Build history of the part. All positions in model axes, mm. A direction names the side the tool comes from. Give positions to 0.01 mm unless a question says otherwise; leave off trailing zeros. Order: outer loops, then holes, each group sorted by start corner. A loop starts at its lowest first (then second) coordinate and runs counter-clockwise, first axis right, second up. Notation, with made-up numbers: (-27, 0) - (-1, 0) arc R22 ccw to (-1, 33) - close; hole circle Ø11 at (43.5, 43.5). An arc over 180 degrees is marked (long way). Answer in a Markdown table with one row per item.
```python
from build123d import *

# Parameters (mm, degrees)
CYLINDER003_R            = 2.65
CYLINDER003_DEPTH        = 9
CLONE009_PLACEMENT_ANGLE = 90
BOX002_W                 = 12
BOX002_H                 = 24
BOX002_DEPTH             = 8
FILLET_R                 = 2
CYLINDER002_R            = 0.925
CYLINDER002_DEPTH        = 7
CYLINDER001_R            = 3
CYLINDER001_DEPTH        = 7
SKETCH002_R              = 1.65
EXTRUDE002_DEPTH         = 3
CLONE010_PLACEMENT_ANGLE = 90


with BuildPart() as insert001:
    # Cylinder003 → Cylinder003 (new body)
    with BuildSketch(Plane(origin=(24, -35, 3), x_dir=(0, 0, 1), z_dir=(-1, 0, 0))):
        Circle(CYLINDER003_R)
    extrude(amount=CYLINDER003_DEPTH)


with BuildPart() as insert002:
    # Clone006 base: copy of insert001
    add(insert001.part)


with BuildPart() as insert002_1:
    # Clone006 placement: moved
    add(insert002.part.moved(Location((0, -16, 0))))


with BuildPart() as obj1:
    # Fusion002 base: copy of insert001
    add(insert001.part)

    # Fusion002: union insert002
    add(insert002_1.part)


with BuildPart() as obj1_1:
    # Fusion002 placement: moved
    add(obj1.part.moved(Location((0, 0, -3))))


with BuildPart() as insertsfusion003:
    # Clone009 base: copy of obj1
    add(obj1_1.part)


with BuildPart() as insertsfusion003_1:
    # Clone009 placement: moved
    add(insertsfusion003.part.moved(Location((0, 50, 62))).rotate(Axis((0, 50, 62), (1, 0, 0)), CLONE009_PLACEMENT_ANGLE))

    # Fusion003: union obj1
    add(obj1_1.part)


with BuildPart() as obj2:
    # Box002 → Box002 (new body)
    with BuildSketch(Plane(origin=(15, -55, -1), x_dir=(1, 0, 0), z_dir=(0, 0, 1))):
        with Locations((6, 12)):
            Rectangle(BOX002_W, BOX002_H)
    extrude(amount=BOX002_DEPTH)

    # Fillet
    fillet_edges = [obj2.edges().sort_by_distance(p)[0] for p in [
        (21, -55, -1),
        (21, -55, 7),
        (21, -31, -1),
        (21, -31, 7),
    ]]
    fillet(fillet_edges, radius=FILLET_R)


with BuildPart() as obj2_1:
    # Fillet placement: moved
    add(obj2.part.moved(Location((0, 0, -3))))


with BuildPart() as hole002:
    # Cylinder002 → Cylinder002 (new body)
    with BuildSketch(Plane(origin=(27, -16, 0), x_dir=(0, 0, 1), z_dir=(-1, 0, 0))):
        Circle(CYLINDER002_R)
    extrude(amount=CYLINDER002_DEPTH)


with BuildPart() as hole003:
    # Clone003 base: copy of hole002
    add(hole002.part)


with BuildPart() as hole003_1:
    # Clone003 placement: moved
    add(hole003.part.moved(Location((0, 0, 36))))


with BuildPart() as hole004:
    # Clone004 base: copy of hole003
    add(hole003_1.part)


with BuildPart() as hole004_1:
    # Clone004 placement: moved
    add(hole004.part.moved(Location((0, 56, -36))))


with BuildPart() as hole005:
    # Clone005 base: copy of hole004
    add(hole004_1.part)


with BuildPart() as hole005_1:
    # Clone005 placement: moved
    add(hole005.part.moved(Location((0, 0, 36))))


with BuildPart() as holesfusion001:
    # Fusion base: copy of hole002
    add(hole002.part)

    # Fusion: union hole003, hole004, hole005
    add(hole003_1.part)
    add(hole004_1.part)
    add(hole005_1.part)


with BuildPart() as attach001:
    # Cylinder001 → Cylinder001 (new body)
    with BuildSketch(Plane(origin=(27, 40, 0), x_dir=(0, 0, 1), z_dir=(-1, 0, 0))):
        Circle(CYLINDER001_R)
    extrude(amount=CYLINDER001_DEPTH)


with BuildPart() as attach002:
    # Clone base: copy of attach001
    add(attach001.part)


with BuildPart() as attach002_1:
    # Clone placement: moved
    add(attach002.part.moved(Location((0, 0, 36))))


with BuildPart() as attach003:
    # Clone001 base: copy of attach002
    add(attach002_1.part)


with BuildPart() as attach003_1:
    # Clone001 placement: moved
    add(attach003.part.moved(Location((0, -56, -36))))


with BuildPart() as attach004:
    # Clone002 base: copy of attach003
    add(attach003_1.part)


with BuildPart() as attach004_1:
    # Clone002 placement: moved
    add(attach004.part.moved(Location((0, 0, 36))))


with BuildPart() as obj3:
    # Sketch002 (on Face5 of Extrude001) → Extrude002 (new body)
    with BuildSketch(Plane.YZ.offset(27)):
        with BuildLine():
            Line((-21.840834, 24.960582), (-53.988857, 12.50779))
            ThreePointArc((-53.988857, 12.50779), (-56.115528, 9.746452), (-54.651077, 6.583683))
            add(Edge.make_bspline(
                [(-54.651077, 6.583683), (-53.010517, 3.198744), (-52.696371, 2.249369), (-51.549184, 1.787077), (-52.006912, 2.204484), (-45.648689, -0.330521), (-21.747141, 0.945049), (-21.747141, 0.945049)],
                knots=[0, 0, 0, 0, 0.2, 0.4, 0.6, 0.8, 1, 1, 1, 1], degree=3))
            ThreePointArc((-21.747141, 0.945049), (-20.257929, 0.297113), (-19.355012, -1.052819))
            ThreePointArc((-19.355012, -1.052819), (-18.192035, -2.749458), (-16.278951, -3.505242))
            Line((-16.278951, -3.505242), (38.983907, -3.505242))
            ThreePointArc((38.983907, -3.505242), (40.694219, -3.582907), (42.251751, -2.872069))
            Line((42.251751, -2.872069), (47.13375, -1.117604))
            ThreePointArc((47.13375, -1.117604), (49.660876, -0.395307), (51.055069, 1.832764))
            Line((51.055069, 1.832764), (49.885408, 38.110058))
            ThreePointArc((49.885408, 38.110058), (50.422789, 40.457526), (52.04587, 42.236569))
            ThreePointArc((52.04587, 42.236569), (53.292041, 46.426402), (49.345321, 48.305506))
            Line((49.345321, 48.305506), (31.159741, 40.29296))
            ThreePointArc((31.159741, 40.29296), (28.834741, 39.544977), (26.405518, 39.292031))
            Line((26.405518, 39.292031), (-15.565081, 39.292031))
            ThreePointArc((-15.565081, 39.292031), (-18.351405, 38.137898), (-19.505538, 35.351575))
            Line((-19.505538, 35.351575), (-19.505538, 28.369553))
            ThreePointArc((-19.505538, 28.369553), (-20.14535, 26.303476), (-21.840834, 24.960582))
        make_face()
        with Locations((-52.774566, 9.372986)):
            Circle(SKETCH002_R, mode=Mode.SUBTRACT)
        with Locations((50.220626, 45.059686)):
            Circle(SKETCH002_R, mode=Mode.SUBTRACT)
        with Locations((46.966619, 2.182986)):
            Circle(SKETCH002_R, mode=Mode.SUBTRACT)
        with BuildLine():
            ThreePointArc((-42.901854, 12.302255), (-43.81194, 10.903698), (-42.6099, 9.746408))
            Line((-42.6099, 9.746408), (41.00829, 3.39546))
            ThreePointArc((41.00829, 3.39546), (44.698125, 5.221862), (46.188436, 9.059779))
            Line((46.188436, 9.059779), (46.188436, 30.650335))
            ThreePointArc((46.188436, 30.650335), (45.602859, 32.064042), (44.189151, 32.649619))
            Line((44.189151, 32.649619), (13.812123, 32.649619))
            Line((13.812123, 32.649619), (-11.694611, 34.281909))
            ThreePointArc((-11.694611, 34.281909), (-13.16559, 33.801037), (-13.900901, 32.439297))
            ThreePointArc((-13.900901, 32.439297), (-13.932701, 32.072334), (-13.943313, 31.704149))
            Line((-13.943313, 31.704149), (-13.943313, 26.615805))
            ThreePointArc((-13.943313, 26.615805), (-14.202233, 24.971619), (-14.953931, 23.48658))
            Line((-14.953931, 23.48658), (-15.353167, 22.932962))
            ThreePointArc((-15.353167, 22.932962), (-16.05756, 22.212579), (-16.942805, 21.731473))
            Line((-16.942805, 21.731473), (-42.901854, 12.302255))
        make_face(mode=Mode.SUBTRACT)
    extrude(amount=-EXTRUDE002_DEPTH)

    # Fusion001: union attach004, attach003, attach002, attach001
    add(attach004_1.part)
    add(attach003_1.part)
    add(attach002_1.part)
    add(attach001.part)

    # Cut001: cut holesFusion001
    add(holesfusion001.part, mode=Mode.SUBTRACT)


with BuildPart() as obj4:
    # Clone010 base: copy of obj2
    add(obj2_1.part)


with BuildPart() as obj4_1:
    # Clone010 placement: moved
    add(obj4.part.moved(Location((0, 50, 62))).rotate(Axis((0, 50, 62), (1, 0, 0)), CLONE010_PLACEMENT_ANGLE))

    # Fusion004: union obj2, obj3
    add(obj2_1.part)
    add(obj3.part)

    # Cut002: cut insertsFusion003
    add(insertsfusion003_1.part, mode=Mode.SUBTRACT)


solid = obj4_1.part
```
1. Two-plate mould, pull along Z, no slides. Class faces 6 (the face through (26, -13.943, 29)), 7 (the face through (25.521, -20.128, 26.329)), 8 (the face through (21.08, -31.57, -3.4)): +Z half, -Z half, draft (parallel to the pull), parting line (faces both ways), or undercut.
Check result:
| item | result |
|---|---|
| face 6 | undercut |
| face 7 | +Z half |
| face 8 | -Z half |
2. Cut at D-D on y = -35. Write the cut outline in (x, z), and give its area (3 significant figures).
Check result:
| item | result |
|---|---|
| outline | (15, -4) - (27, -4) - (27, 9.17) - (24, 9.17) - (24, 4) - (15, 4) - (15, 2.65) - (24, 2.65) - (24, -2.65) - (15, -2.65) - close; (24, 15.17) - (27, 15.17) - (27, 19.86) - (24, 19.86) - close |
| area | 77.9 mm² |
3. Drop flat-ended pins along their axis: P1, Ø6.5, axis at y = 40, z = 35.5, coming from the -X side; P2, Ø4, axis at x = 16.5, z = 21, coming from the -Y side; P3, Ø0.9, axis at x = 25.5, z = 30, coming from the -Y side; P4, Ø4.5, axis at y = -52.77, z = 9.37, coming from the +X side. Give the stop position or say it passes through.
Check result:
| item | result |
|---|---|
| P1 | stops at x = 20 |
| P2 | stops at y = 46 |
| P3 | stops at y = -19.51 |
| P4 | stops at x = 27 |
4. Which spindle directions (+Z, -Z, +X, -X, +Y, -Y) get a long thin tool onto all of the face, cutting with end or side? Do faces 1 (the face through (21, 46, 19)), 2 (the face through (25.521, -20.276, 0.312)), 3 (the face through (24, 50, 11)), 4 (the face through (26, -19.506, 32)), 5 (the face through (21.08, 53.4, 30.43)). Say none if no direction does.
Check result:
| item | result |
|---|---|
| face 1 | +X, -X |
| face 2 | -Z, +X, -X |
| face 3 | -X |
| face 4 | +Z, +X, -X, -Y |
| face 5 | +X, -X, +Y |
5. Cut at B-B on x = 22.25. Count the separate pieces of the cut face and the enclosed holes in it, and give its area (3 significant figures).
Check result:
| item | result |
|---|---|
| separate pieces | 6 |
| enclosed holes | 8 |
| area | 391 mm² |
6. Cut at A-A on x = 16.25. Write the cut outline in (y, z), and give its area (3 significant figures).
Check result:
| item | result |
|---|---|
| outline | (-55, -2) arc R2 ccw to (-53, -4) - (-33, -4) arc R2 ccw to (-31, -2) - (-31, 2) arc R2 ccw to (-33, 4) - (-53, 4) arc R2 ccw to (-55, 2) - close; (46, 9) arc R2 ccw to (48, 7) - (52, 7) arc R2 ccw to (54, 9) - (54, 29) arc R2 ccw to (52, 31) - (48, 31) arc R2 ccw to (46, 29) - close; hole circle Ø5.3 at (-51, 0); hole circle Ø5.3 at (-35, 0); hole circle Ø5.3 at (50, 11); hole circle Ø5.3 at (50, 27) |
| area | 289 mm² |
7. Cut at C-C on z = 17. Write the cut outline in (x, y).
Check result:
| item | result |
|---|---|
| outline | (15, 46) - (27, 46) - (27, 54) - (15, 54) - close; (24, -42.39) - (27, -42.39) - (27, -29.97) - (24, -29.97) - close |
8. Probe line 1 (Z direction, x = 22, y = 40) (3 decimals); line 2 (Y direction, x = 23.75, z = 36) (3 decimals); line 3 (Z direction, x = 20.5, y = 50). List the from-to ranges inside material, lowest first.
Check result:
| item | result |
|---|---|
| line 1 | z = -3 to -0.925, 0.925 to 3, 33 to 35.075, 36.925 to 39 |
| line 2 | y = -19 to -16.925, -15.075 to -13, 37 to 39.075, 40.925 to 43 |
| line 3 | z = 7 to 8.35, 13.65 to 24.35, 29.65 to 31 |
